Input: part model. Units: mm. Frame: model coordinates. A direction names the side the tool comes from. Round coordinates to 2 decimals unless told otherwise and drop trailing zeros. Loops run counter-clockwise (first coordinate to the right, second up) from the corner with the lowest first, then second, coordinate; pieces in that order, holes last. Notation, with made-up numbers: (15.25, -8) -> (32.25, -8) arc R25 cw to (32.25, 16) -> close; hole circle Ø3 at (56, -20.5). An arc over 180 degrees is marked (long way). Answer as a JSON object with one key per item and string values. Group by question number.
Item 1: Material intervals for line 1 (Y direction, x = -15.6, z = -58); line 2 (X direction, y = -3.5, z = -74); line 3 (Z direction, x = -13.8, y = 0), sorted ascending. Write a range as [from, to].
Item 2: Section query B-B on x = -3.5. Return loops of the section in (y, z).
Item 3: Section query C-C on z = -24. Return loops of the section in (x, y), and give its area (3 significant figures).
Item 4: Pin query (flat end, axial travel): pin 1 (5 mm diameter, centred on y = 3.5, z = -16, fed in from -X); pin 2 (3 mm diameter, centred on y = 1, z = -6, fed in from -X); pin 3 (2.5 mm diameter, centred on y = 0, z = -58, fed in from +X); pin 4 (4 mm diameter, centred on y = -2, z = -37, fed in from +X). Return the tip coordinate at first contact, or that it passes through.
Item 5: Set-up query: faces 4 (the flat face through (-6, 0, -5)), 5 (the cylindrical face through (0.507, 3.905, -4.133)), 6 (the flat face through (-12.5, 0, -61)), 7 (the flat face through (-8.62, 0.07, -35.07)). Return all of +Z, -Z, +X, -X, +Y, -Y with unobstructed straight access to the full face (end or side cutting, diameter ignored); none if empty.
Item 6: Draft query along Y for faces 1 (the cylindrical face through (-14.781, 0.481, -59.526)), 2 (the cylindrical face through (-3, 0, -2)), 3 (the flat face through (-8, -5, -40)). Return one class per face: released by +Y, released by -Y, zero draft, split by the parting line, or undercut.
Item 7: Section query A-A on z = -48. Return loops of the section in (x, y).
from build123d import *

# Parameters (mm, degrees)
EXTRUDE_2_DEPTH          = 5
CUT_EXTRUDE_1_DEPTH      = 83.044195407
CUT_EXTRUDE_1_DEPTH_BACK = 83.044195407
SKETCH_3_OUTSIDE_W       = 98.714
SKETCH_3_OUTSIDE_H       = 28.714
CUT_EXTRUDE_2_DEPTH      = 84.120394609
CUT_EXTRUDE_2_DEPTH_BACK = 84.120394609
SKETCH_4_R               = 1.6
SKETCH_5_R               = 3
EXTRUDE_4_DEPTH          = 6
CUT_EXTRUDE_3_DEPTH      = 82.939001702
CUT_EXTRUDE_3_DEPTH_BACK = 1
SKETCH_6_R               = 4


with BuildPart() as part:
    # 草图2 → 凸台-拉伸2 (new, symmetric)
    with BuildSketch(Plane(origin=(0, 0, 0), x_dir=(1, 0, 0), z_dir=(0, 1, 0))):
        Polygon((-17, 40), (0, 30), (0, 0), (5, 0), (5, 32.859730272), (-12.5, 43.153847919), (-12.5, 80), (-17, 80), align=None)
    extrude(amount=EXTRUDE_2_DEPTH, both=True)

    # 草图3 outside → 切除-拉伸1 (cut, two sides: drawn at the far end of the back side and taken through both)
    with BuildSketch(Plane(origin=(-12.5, 0, 0), x_dir=(0, 0, -1), z_dir=(1, 0, 0)).offset(-CUT_EXTRUDE_1_DEPTH_BACK)):
        with Locations((40, 0)):
            Rectangle(SKETCH_3_OUTSIDE_W, SKETCH_3_OUTSIDE_H)
        with BuildLine():
            Line((5, 5), (75, 5))
            ThreePointArc((75, 5), (80, 0), (75, -5))
            Line((75, -5), (5, -5))
            ThreePointArc((5, -5), (0, 0), (5, 5))
        make_face(mode=Mode.SUBTRACT)
    extrude(amount=CUT_EXTRUDE_1_DEPTH + CUT_EXTRUDE_1_DEPTH_BACK, mode=Mode.SUBTRACT)

    # 草图4 → 切除-拉伸2 (cut, two sides: drawn at the far end of the back side and taken through both)
    with BuildSketch(Plane(origin=(5, 0, 0), x_dir=(0, 0, -1), z_dir=(1, 0, 0)).offset(-CUT_EXTRUDE_2_DEPTH_BACK)):
        with Locations((75, 0)):
            Circle(SKETCH_4_R)
        with Locations((58, 0)):
            Circle(SKETCH_4_R)
        with Locations((48, 0)):
            Circle(SKETCH_4_R)
    extrude(amount=CUT_EXTRUDE_2_DEPTH + CUT_EXTRUDE_2_DEPTH_BACK, mode=Mode.SUBTRACT)

    # 草图5 → 凸台-拉伸4 (add)
    with BuildSketch(Plane.ZY):
        with Locations(Location((-5, 0, 0), (0, 0, 180))):
            Circle(SKETCH_5_R)
    extrude(amount=EXTRUDE_4_DEPTH)

    # 草图6 → 切除-拉伸3 (cut, two sides: drawn at the far end of the back side and taken through both)
    with BuildSketch(Plane.ZY.offset(-CUT_EXTRUDE_3_DEPTH_BACK)):
        with BuildLine():
            Line((-5, 5), (-30, 5))
            Line((-30, 5), (-30, -5))
            Line((-30, -5), (-5, -5))
            ThreePointArc((-5, -5), (0, 0), (-5, 5))
        make_face()
        with Locations(Location((-5, 0, 0), (0, 0, 180))):
            Circle(SKETCH_6_R, mode=Mode.SUBTRACT)
    extrude(amount=CUT_EXTRUDE_3_DEPTH + CUT_EXTRUDE_3_DEPTH_BACK, mode=Mode.SUBTRACT)


solid = part.part
Solved:
{
 "1": {"line 1": "[-5, -1.6], [1.6, 5]", "line 2": "[-17, -12.5]", "line 3": "[-80, -76.6], [-73.4, -59.6], [-56.4, -49.6], [-46.4, -38.12]"},
 "2": {"outline": "(-5, -37.86) -> (5, -37.86) -> (5, -32.06) -> (-5, -32.06) -> close; circle Ø6 at (0, -5)"},
 "3": {"outline": "(1, -5) -> (5, -5) -> (5, 5) -> (1, 5) -> close", "area": "40.0 mm²"},
 "4": {"pin 1": "x = 1", "pin 2": "x = -6", "pin 3": "through", "pin 4": "x = 1.36"},
 "5": {"face 4": "+Z, -X, +Y, -Y", "face 5": "-X", "face 6": "-Z, +X, +Y, -Y", "face 7": "-X, +Y, -Y"},
 "6": {"face 1": "undercut", "face 2": "split by the parting line", "face 3": "released by -Y"},
 "7": {"outline": "(-17, -5) -> (-12.5, -5) -> (-12.5, -1.6) -> (-17, -1.6) -> close; (-17, 1.6) -> (-12.5, 1.6) -> (-12.5, 5) -> (-17, 5) -> close"}
}
